from build123d import *

# Parameters (mm, degrees)
CYLINDER004_R            = 3
CYLINDER004_DEPTH        = 10
PAD010_DEPTH             = 10
SKETCH036_R              = 1.75
POCKET025_DEPTH          = 45.001
CHAMFER023_1_SIZE        = 3
CHAMFER023_2_SIZE        = 2
CHAMFER023_3_SIZE        = 1
CHAMFER024_SIZE          = 0.5
CLONE007_PITCH_ANGLE     = 90
CLONE007_PLACEMENT_ANGLE = 45


with BuildPart() as boardbracketscrewheadcylinder001:
    # Cylinder004 → Cylinder004 (new body)
    with BuildSketch(Plane(origin=(0, 0.5, 24), x_dir=(1, 0, 0), z_dir=(0, 0, 1))):
        Circle(CYLINDER004_R)
    extrude(amount=CYLINDER004_DEPTH)


with BuildPart() as clone007:
    # Sketch035 → Pad010 (new body, symmetric)
    with BuildSketch(Plane.YZ):
        Polygon((4.5, 21), (4.5, 24), (-0.12132, 28.62132), (-5.071068, 33.571068), (-7.545942, 31.096194), (-6.838835, 30.389087), (-5.778175, 31.449747), (-4.717514, 30.389087), (-6.131728, 28.974874), (-2.949747, 25.792893), (-35.476659, -6.734019), (-38.65864, -3.552038), (-40.072853, -4.966252), (-41.133514, -3.905592), (-40.072853, -2.844931), (-40.77996, -2.137825), (-43.254834, -4.612698), (-38.305087, -9.562446), (-36.183766, -11.683766), (-25.12132, -0.62132), (-4.742641, -21), (4.5, -21), (4.5, -18), (-3.5, -18), (-23, 1.5), (-3.5, 21), align=None)
    extrude(amount=PAD010_DEPTH, both=True)

    # Cut002: cut BoardBracketScrewHeadCylinder001
    add(boardbracketscrewheadcylinder001.part, mode=Mode.SUBTRACT)

    # Sketch036 → Pocket025 (cut, through all)
    with BuildSketch(Plane.XY.offset(24)):
        with Locations((0, 0.5)):
            Circle(SKETCH036_R)
    extrude(amount=-POCKET025_DEPTH, mode=Mode.SUBTRACT)

    # Chamfer023 1
    chamfer023_1_edges = [clone007.edges().sort_by_distance(p)[0] for p in [
        (0, -36.183766, -11.683766),
    ]]
    chamfer(chamfer023_1_edges, length=CHAMFER023_1_SIZE)

    # Chamfer023 2
    chamfer023_2_edges = [clone007.edges().sort_by_distance(p)[0] for p in [
        (0, -25.12132, -0.62132),
    ]]
    chamfer(chamfer023_2_edges, length=CHAMFER023_2_SIZE)

    # Chamfer023 3
    chamfer023_3_edges = [clone007.edges().sort_by_distance(p)[0] for p in [
        (0, -35.476659, -6.734019),
        (0, -43.254834, -4.612698),
        (0, -5.071068, 33.571068),
    ]]
    chamfer(chamfer023_3_edges, length=CHAMFER023_3_SIZE)

    # Chamfer024
    chamfer024_edges = [clone007.edges().sort_by_distance(p)[0] for p in [
        (10, -5.424621, 29.681981),
        (10, -39.365747, -4.259145),
        (10, -5.247845, 30.919417),
        (10, -40.603184, -4.435922),
        (10, 4.5, 22.5),
        (10, 0.5, 21),
        (10, -13.25, 11.25),
        (10, -13.25, -8.25),
        (10, 0.5, -18),
        (10, 4.5, -19.5),
    ]]
    chamfer(chamfer024_edges, length=CHAMFER024_SIZE)


with BuildPart() as clone007_1:
    # Clone007 pitch: moved
    add(clone007.part.rotate(Axis((0, 0, 0), (0, 1, 0)), CLONE007_PITCH_ANGLE))


with BuildPart() as clone007_2:
    # Clone007 placement: moved
    add(clone007_1.part.moved(Location((-220.999994, 1.999983, -27.49999))).rotate(Axis((-220.999994, 1.999983, -27.49999), (0, 0, 1)), CLONE007_PLACEMENT_ANGLE))


solid = clone007_2.part
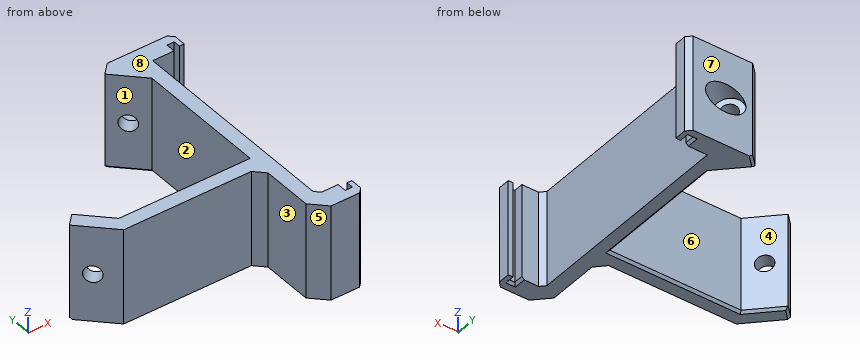
Can you work these out from the model? Positions are in its coordinate system, mm. Face numbers are marked on the shaded views. A direction names the side the tool comes from. Round coordinates to 2 decimals unless told otherwise and drop trailing zeros. Loops run counter-clockwise (first coordinate to the right, second up) from the corner with the lowest first, then second, coordinate; pieces in that order, holes last. Notation, with made-up numbers: (60, -13.75) - (113, -13.75) arc R22 cw to (113, 22.25) - close; hole circle Ø5 at (76.5, -7.75). An arc over 180 degrees is marked (long way). Answer in a Markdown table with one row per item. Add a question column.
Q1. We'd pull the mould along Y, two halves only. Please class the marked faces 5, 6, 7 and 8: pulls with the +Y half, pulls with the -Y half, needs draft (parallel to the pull), parting line crosses it, or undercut.
Q2. Which directions (+Z, -Z, +X, -X, +Y, -Y) give clear straight access to the entire face, cutting with the end or side of a thin tool? Please do the marked faces 1, 2, 3 and 4.
Q3. I need wall thicknesses on L1, parallel to Y at x = -199, z = -32.75; L2, parallel to X at y = 6, z = -24; L3, parallel to X at y = -10, z = -32.5. Which ranges of each line are inside material? Lowest first, please.
Q4. I want a section at C-C on x = -221. List the corners of the cut face in (y, z) for me, and give its area (3 significant figures).
Q5. I want a section at B-B on y = 3. List the corners of the cut face in (x, z) for me, and give its area (3 significant figures).
Q6. I want a section at D-D on z = -28.5. Count the separate pieces of the cut face and the enclosed holes in it, and give its area (3 significant figures).
Q7. For pin 1 Ø5.5 at (y, z) = (-24, -23.5) entering from -X; pin 2 Ø6 at (y, z) = (13, -23) entering from -X; pin 3 Ø6 at (y, z) = (-9.5, -31) entering from +X, each with a flat end and sliding along its axis, tell me the tip position at first contact or that it passes through.
A:
| question | item | result |
|---|---|---|
| 1 | face 5 | pulls with the -Y half |
| 1 | face 6 | undercut |
| 1 | face 7 | pulls with the +Y half |
| 1 | face 8 | needs draft |
| 2 | face 1 | +Z, -Z, -X |
| 2 | face 2 | +Z, -Z |
| 2 | face 3 | +Z, -Z, -X, -Y |
| 2 | face 4 | +Z, -Z, +Y |
| 3 | L1 | -31.85 to -27.85, 18.15 to 22.15 |
| 3 | L2 | -203.68 to -200.68 |
| 3 | L3 | -238.7 to -234.46, -203.68 to -200.68 |
| 4 | outline | (-16.2, -37.5) - (-13.7, -37.5) - (-13.2, -37) - (-13.2, -17.5) - (-16.2, -17.5) - close |
| 4 | area | 59.9 mm^2 |
| 5 | outline | (-203.68, -37) - (-203.18, -37.5) - (-200.68, -37.5) - (-200.68, -17.5) - (-203.68, -17.5) - close |
| 5 | area | 59.9 mm^2 |
| 6 | separate pieces | 3 |
| 6 | enclosed holes | 0 |
| 6 | area | 304 mm^2 |
| 7 | pin 1 | x = -203.68 |
| 7 | pin 2 | x = -205.3 |
| 7 | pin 3 | x = -200.68 |
